Geometry check sheet. Reference: the model listing, model coordinates, mm. Face numbers are marked on the shaded views. Coordinates: 2 decimals unless noted, no trailing zeros. Loops run counter-clockwise (first coordinate to the right, second up) from the corner with the lowest first, then second, coordinate; pieces in that order, holes last.
from build123d import *

# Parameters (mm, degrees)
SKETCH1_R           = 8
BOSS_EXTRUDE1_DEPTH = 24
SKETCH2_R           = 10
BOSS_EXTRUDE2_DEPTH = 3
SKETCH4_R           = 8
SKETCH4_R_2         = 7.6
CUT_EXTRUDE1_DEPTH  = 1.2
SKETCH5_R           = 6.2
CUT_EXTRUDE2_DEPTH  = 25
CHAMFER1_SIZE       = 0.4
CHAMFER2_SIZE       = 0.4


with BuildPart() as part:
    # Sketch1 → Boss-Extrude1 (new body)
    with BuildSketch(Plane(origin=(0, 0, 0), x_dir=(1, 0, 0), z_dir=(0, 1, 0))):
        Circle(SKETCH1_R)
    extrude(amount=BOSS_EXTRUDE1_DEPTH)

    # Sketch2 → Boss-Extrude2 (add)
    with BuildSketch(Plane.XZ):
        Circle(SKETCH2_R)
    extrude(amount=-BOSS_EXTRUDE2_DEPTH)

    # Sketch4 → Cut-Extrude1 (cut)
    with BuildSketch(Plane(origin=(0, 20, 0), x_dir=(1, 0, 0), z_dir=(0, 1, 0))):
        Circle(SKETCH4_R)
        Circle(SKETCH4_R_2, mode=Mode.SUBTRACT)
    extrude(amount=CUT_EXTRUDE1_DEPTH, mode=Mode.SUBTRACT)

    # Sketch5 → Cut-Extrude2 (cut, through all)
    with BuildSketch(Plane.XZ):
        Circle(SKETCH5_R)
    extrude(amount=-CUT_EXTRUDE2_DEPTH, mode=Mode.SUBTRACT)

    # Chamfer1
    chamfer1_edges = [part.edges().sort_by_distance(p)[0] for p in [
        (-6.2, 24, 0),
        (-6.2, 0, 0),
    ]]
    chamfer(chamfer1_edges, length=CHAMFER1_SIZE)

    # Chamfer2
    chamfer2_edges = [part.edges().sort_by_distance(p)[0] for p in [
        (-8, 24, 0),
        (-10, 3, 0),
        (-10, 0, 0),
    ]]
    chamfer(chamfer2_edges, length=CHAMFER2_SIZE)


solid = part.part
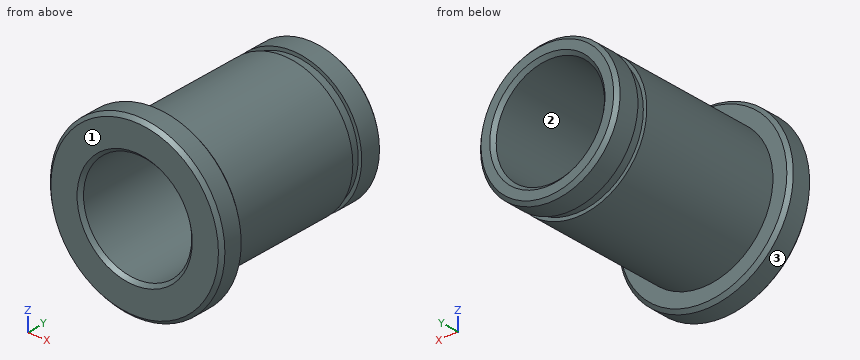
(1) Sectioned sample at C-C on y = 17.5. Record the cut outline in (x, z), and give its area (3 significant figures).
Findings:
outline: circle Ø16 at (0, 0); hole circle Ø12.4 at (0, 0)
area: 80.3 mm2
(2) Draft check along Z on the marked faces 1, 2 and 3. Enter one of: +Z half, -Z half, draft (parallel to the pull), parting line (faces both ways), or undercut.
Findings:
face 1: draft
face 2: undercut
face 3: parting line
(3) Gauge pin test, flat ends, axial feed: pin 1 Ø10 at (x, y) = (0, 17) entering from -Z; pin 2 Ø5 at (x, z) = (-2.5, -1) entering from -Y; pin 3 Ø6 at (x, y) = (-3.5, 15) entering from +Z; pin 4 Ø1 at (y, z) = (18, -5) entering from -X. Record the tip position at first contact, or that the pin passes through.
Findings:
pin 1: stops at z = -8
pin 2: passes through
pin 3: stops at z = 7.98
pin 4: stops at x = -6.61
(4) Scan lines: L1, parallel to Z at x = 0, y = 10.25; L2, parallel to Y at x = -3.25, z = -8.25; L3, parallel to Z at x = 4.5, y = 17.25. Record each from-to range of solid material in increasing order.
Findings:
L1: z = -8 to -6.2, 6.2 to 8
L2: y = 0 to 3
L3: z = -6.61 to -4.26, 4.26 to 6.61
